from build123d import *

# Parameters (mm, degrees)
SKETCH1_R           = 1.25
BOSS_EXTRUDE1_DEPTH = 60
FILLET1_R           = 1


with BuildPart() as part:
    # Sketch1 → Boss-Extrude1 (new body)
    with BuildSketch(Plane.XY):
        Polygon((7.5, -7.5), (1.7, -7.5), (1.7, -6.4), (2.85, -6.4), (2.85, -3.63183498), (2.01816502, -2.8), (-2.01816502, -2.8), (-2.85, -3.63183498), (-2.85, -6.4), (-1.7, -6.4), (-1.7, -7.5), (-7.5, -7.5), (-7.5, -1.7), (-6.4, -1.7), (-6.4, -2.85), (-3.63183498, -2.85), (-2.8, -2.01816502), (-2.8, 2.01816502), (-3.63183498, 2.85), (-6.4, 2.85), (-6.4, 1.7), (-7.5, 1.7), (-7.5, 7.5), (-1.7, 7.5), (-1.7, 6.4), (-2.85, 6.4), (-2.85, 3.63183498), (-2.01816502, 2.8), (2.01816502, 2.8), (2.85, 3.63183498), (2.85, 6.4), (1.7, 6.4), (1.7, 7.5), (7.5, 7.5), (7.5, 1.7), (6.4, 1.7), (6.4, 2.85), (3.63183498, 2.85), (2.8, 2.01816502), (2.8, -2.01816502), (3.63183498, -2.85), (6.4, -2.85), (6.4, -1.7), (7.5, -1.7), align=None)
        Circle(SKETCH1_R, mode=Mode.SUBTRACT)
    extrude(amount=BOSS_EXTRUDE1_DEPTH)

    # Fillet1
    fillet1_edges = [part.edges().sort_by_distance(p)[0] for p in [
        (-7.5, 7.5, 30),
        (7.5, 7.5, 30),
        (7.5, -7.5, 30),
        (-7.5, -7.5, 30),
    ]]
    fillet(fillet1_edges, radius=FILLET1_R)


solid = part.part
Can you work these out from the model? Positions are in its coordinate system, mm. A direction names the side the tool comes from. Give positions to 0.01 mm unless a question says otherwise; leave off trailing zeros. Loops run counter-clockwise (first coordinate to the right, second up) from the corner with the lowest first, then second, coordinate; pieces in that order, holes last. Notation, with made-up numbers: (-36, -3.75) - (-5, -3.75) arc R28 cw to (-5, 28.25) - close; hole circle Ø8 at (-33, -27.5). An arc over 180 degrees is marked (long way). One line per item, written item: value.
(1) I need wall thicknesses on line 1 along X through (y, z) = (2, 17.5); line 2 along Y through (x, z) = (-4.75, 30.5). Which ranges of each line are inside material? Lowest first, please.
Verdict:
line 1: -7.5 to -6.4, -2.8 to 2.8, 6.4 to 7.5
line 2: -7.5 to -2.85, 2.85 to 7.5
(2) If we mould it in two halves opening along Y, with no side actions, what happens to faces 1 (the face through (0, 2, 0)), 2 (the face through (5, -2.85, 30)), 3 (the face through (-7.215, 7.199, 30.42))? For each: released by +Y, released by -Y, zero draft, split by the parting line, or undercut.
Verdict:
face 1: zero draft
face 2: undercut
face 3: released by +Y
(3) I'm going to push flat-ended pins straight in: pin 1 (1 mm diameter, centred on y = 0, z = 50, fed in from -X); pin 2 (1.5 mm diameter, centred on x = -5.5, y = -1, fed in from -Z); pin 3 (2 mm diameter, centred on y = 0.5, z = 41.5, fed in from +X). Where does each tip first touch, or does it pass through?
Verdict:
pin 1: x = -2.8
pin 2: through
pin 3: x = 2.8
(4) If we section it at B-B, the plane x = -4.25: List the corners of the cut face in (y, z) for me.
Verdict:
outline: (-7.5, 0) - (-2.85, 0) - (-2.85, 60) - (-7.5, 60) - close; (2.85, 0) - (7.5, 0) - (7.5, 60) - (2.85, 60) - close
(5) If we section it at A-A, the plane y = 0: List the corners of the cut face in (x, z) for me.
Verdict:
outline: (-2.8, 0) - (-1.25, 0) - (-1.25, 60) - (-2.8, 60) - close; (1.25, 0) - (2.8, 0) - (2.8, 60) - (1.25, 60) - close
(6) On a 3-axis mill with a long thin cutter (end or side, diameter ignored), from which of +Z, -Z, +X, -X, +Y, -Y can I reach the whole of each face in a straight line? I mean faces 4 (the face through (1.7, -7, 30)), 5 (the face through (1.7, 7, 30)), 6 (the face through (7.5, 4, 30)), 7 (the face through (2.8, 0, 30)), 8 (the face through (-4, -7.5, 30)). Say none if no direction works.
Verdict:
face 4: +Z, -Z, -Y
face 5: +Z, -Z, +Y
face 6: +Z, -Z, +X, +Y, -Y
face 7: +Z, -Z
face 8: +Z, -Z, +X, -X, -Y
